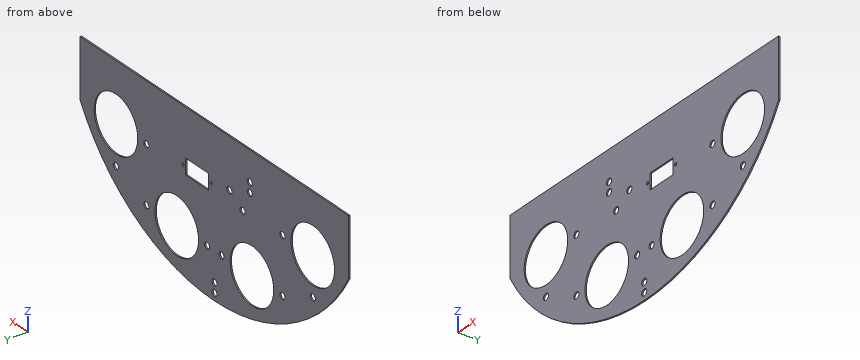
```python
from build123d import *

# Parameters (mm, degrees)
SKETCH3_R             = 21.5
BOSS_EXTRUDE3_DEPTH   = 1
F_5_0MM_DOWEL_HOLE1_D = 5
SKETCH10_R            = 2.5
SKETCH10_R_2          = 1.1
CUT_EXTRUDE3_DEPTH    = 170.731914631


with BuildPart() as part:
    # Sketch3 → Boss-Extrude3 (new body)
    with BuildSketch(Plane(origin=(0, 0, 0), x_dir=(1, 0, 0), z_dir=(0, 1, 0))):
        with BuildLine():
            Line((-132.226234517, -18.972612677), (132.537224892, -18.972612677))
            Line((132.537224892, -18.972612677), (132.537224892, 26.561617598))
            ThreePointArc((132.537224892, 26.561617598), (0.155495187, 106.027387323), (-132.226234517, 26.561617598))
            Line((-132.226234517, 26.561617598), (-132.226234517, -18.972612677))
        make_face()
        with Locations(Location((-96.926544138, 26.561617598, 0), (0, 0, 270))):
            Circle(SKETCH3_R, mode=Mode.SUBTRACT)
        with Locations(Location((97.237534512, 26.561617598, 0), (0, 0, 270))):
            Circle(SKETCH3_R, mode=Mode.SUBTRACT)
        with Locations(Location((-36.926544138, 70.154169278, 0), (0, 0, 270))):
            Circle(SKETCH3_R, mode=Mode.SUBTRACT)
        with Locations(Location((37.237534512, 70.154169278, 0), (0, 0, 270))):
            Circle(SKETCH3_R, mode=Mode.SUBTRACT)
    extrude(amount=BOSS_EXTRUDE3_DEPTH)

    # Ø5.0mm Dowel Hole1 (through all)
    with Locations(Plane(origin=(0, 0, 0), x_dir=(-1, 0, 0), z_dir=(0, -1, 0))):
        with Locations((-97.237534512, 56.561617598), (-67.237534512, 26.561617598), (-67.237534512, 70.154169278), (-7.237534512, 70.154169278), (6.926544138, 70.154169278), (66.926544138, 70.154169278), (96.926544138, 56.561617598), (66.926544138, 26.561617598)):
            Hole(F_5_0MM_DOWEL_HOLE1_D / 2)

    # Sketch10 → Cut-Extrude3 (cut, through all)
    with BuildSketch(Plane(origin=(0, 0, 0), x_dir=(-1, 0, 0), z_dir=(0, -1, 0))):
        Polygon((-28.426423082, 29.82316033), (-28.426423082, 17.62316033), (-16.520871415, 17.62316033), (-5.926423082, 17.62316033), (-5.926423082, 29.82316033), align=None)
        with Locations(Location((27.687865217, 28.254616687, 0), (0, 0, 90))):
            Circle(SKETCH10_R)
        with Locations(Location((14.700079453, 19.79486368, 0), (0, 0, 90))):
            Circle(SKETCH10_R)
        with Locations(Location((34.747097156, 11.87316033, 0), (0, 0, 90))):
            Circle(SKETCH10_R)
        with Locations(Location((34.747097156, 4.37316033, 0), (0, 0, 90))):
            Circle(SKETCH10_R)
        with Locations(Location((-0.03130886, 92.861330123, 0), (0, 0, 90))):
            Circle(SKETCH10_R)
        with Locations(Location((-0.026423082, 100.361328532, 0), (0, 0, 90))):
            Circle(SKETCH10_R)
        with Locations(Location((-31.076423082, 23.72316033, 0), (0, 0, 90))):
            Circle(SKETCH10_R_2)
        with Locations(Location((-3.276423082, 23.72316033, 0), (0, 0, 90))):
            Circle(SKETCH10_R_2)
    extrude(amount=-CUT_EXTRUDE3_DEPTH, mode=Mode.SUBTRACT)


solid = part.part
```
Build history of the part. All positions in model axes, mm. Give positions to 0.01 mm unless a question says otherwise; leave off trailing zeros. Loops run counter-clockwise (first coordinate to the right, second up) from the corner with the lowest first, then second, coordinate; pieces in that order, holes last. Notation, with made-up numbers: (2, -1.5) - (7, -1.5) arc R17 ccw to (7, 4.5) - close; hole circle Ø4 at (27, 26). An arc over 180 degrees is marked (long way). Use a Markdown table: item, result.
(1) Band-saw the part on A-A (z = -34). Give the cut face in (x, y).
Taken from the geometry:
| item | result |
|---|---|
| outline | (-127.99, 0) - (-117.1, 0) - (-117.1, 1) - (-127.99, 1) - close; (-76.75, 0) - (77.07, 0) - (77.07, 1) - (-76.75, 1) - close; (117.41, 0) - (128.3, 0) - (128.3, 1) - (117.41, 1) - close |
(2) Band-saw the part on D-D (z = -75). Give the cut face in (x, y), and give its area (3 significant figures).
Taken from the geometry:
| item | result |
|---|---|
| outline | (-91.2, 0) - (-57.87, 0) - (-57.87, 1) - (-91.2, 1) - close; (-15.98, 0) - (16.29, 0) - (16.29, 1) - (-15.98, 1) - close; (58.18, 0) - (91.51, 0) - (91.51, 1) - (58.18, 1) - close |
| area | 98.9 mm2 |
(3) Wall check: line 1 along Z through (x, y) = (95.5, 0.8); line 2 along X through (y, z) = (0.8, -62); line 3 along X through (y, z) = (0.75, -54). Give the ranges that are in metal, low to high.
Taken from the geometry:
| item | result |
|---|---|
| line 1 | -71.83 to -58.36, -54.76 to -47.99, -5.13 to 18.97 |
| line 2 | -106 to -56.82, -17.03 to 17.34, 57.13 to 106.31 |
| line 3 | -113.43 to -51.11, -22.74 to 23.05, 51.43 to 113.74 |
(4) Band-saw the part on C-C (y = 0.2). Give the number of separate pieces and of enclosed holes in the cut face, and give its area (3 significant figures).
Taken from the geometry:
| item | result |
|---|---|
| separate pieces | 1 |
| enclosed holes | 21 |
| area | 20,700 mm2 |
(5) Band-saw the part on B-B (x = -104). Give the cut face in (y, z).
Taken from the geometry:
| item | result |
|---|---|
| outline | (0, -63.97) - (1, -63.97) - (1, -46.86) - (0, -46.86) - close; (0, -6.26) - (1, -6.26) - (1, 18.97) - (0, 18.97) - close |
(6) Drop a flat-ended pin along its axis: pin 1 Ø4.5 at (x, z) = (-34.75, -4.37) entering from +Y. Give the stop position or say it passes through.
Taken from the geometry:
| item | result |
|---|---|
| pin 1 | through |
